Work out the finished part from the listing and answer in its coordinate system (mm). A direction names the side the tool comes from. Coordinates: 2 decimals unless noted, no trailing zeros. Order: outer loops, then holes, each group sorted by start corner. A loop starts at its lowest first (then second) coordinate and runs counter-clockwise, first axis right, second up. Notation, with made-up numbers: M -16,4.5 L 11,4.5 A27 cw 11,32.5 Z; hole C -6,81 d8. An arc over 180 degrees is marked long. Answer in a Markdown table with one row per item. Add a question column.
Item 1: The mould has two halves that part along X. Classify faces 3 (the face through (-10.79, 46, 1.24)), 4 (the face through (-10.91, 46.94, 2.96)), 5 (the face through (-11.246, 34.387, 0.246)), 6 (the face through (-13, 46, 6)): released by +X, released by -X, zero draft, split by the parting line, or undercut.
Item 2: The part is cut by section D-D (z = 0.85). Write down the section's boundary in (x, y), then the cut area to 3 significant figures.
Item 3: Consider line 1 (Y direction, x = -10, z = 3.65); line 2 (Y direction, x = -10, z = 0.3); line 3 (X direction, y = 35.75, z = 2.45). Determine where each line is inside the solid, lowest interval first. Write a range as from..to.
Item 4: The part is cut by section A-A (x = -10). Write down the section's boundary in (y, z).
Item 5: Flat-ended cylindrical pins translate along their axes: pin 1 Ø7 at (x, y) = (-10, 40) entering from -Z (3 decimals); pin 2 Ø1.5 at (x, z) = (-11.5, 2.5) entering from +Y; pin 3 Ø1 at (y, z) = (44, 2) entering from +X; pin 4 Ø1.5 at (x, y) = (-14.5, 42.5) entering from +Z. Find the tip coordinate at first contact, or state that the pin passes through.
Item 6: Which of the six approach directions +Z, -Z, +X, -X, +Y, -Y give full straight-line access (tool end or side, diameter ignored) to faces 1 (the face through (-10.8, 46.2, 4)), 2 (the face through (-11, 46, 0))?
Item 7: The part is cut by section C-C (z = 4.3). Write down the section's boundary in (x, y).
Item 8: The part is cut by section B-B (y = 40). Write down the section's boundary in (x, z).
from build123d import *

# Parameters (mm, degrees)
CYLINDER011_R     = 6.25
CYLINDER011_DEPTH = 10
CYLINDER010_R     = 6.05
CYLINDER010_DEPTH = 10
CYLINDER009_R     = 5.75
CYLINDER009_DEPTH = 10
CYLINDER008_R     = 7
CYLINDER008_DEPTH = 6


with BuildPart() as bluetmp06:
    # Cylinder011 → Cylinder011 (new body)
    with BuildSketch(Plane.XY.offset(2)):
        Circle(CYLINDER011_R)
    extrude(amount=CYLINDER011_DEPTH)


with BuildPart() as bluetmp04:
    # Cylinder010 → Cylinder010 (new body)
    with BuildSketch(Plane.XY.offset(0.5)):
        Circle(CYLINDER010_R)
    extrude(amount=CYLINDER010_DEPTH)


with BuildPart() as bluetmp02:
    # Cylinder009 → Cylinder009 (new body)
    with BuildSketch(Plane.XY):
        Circle(CYLINDER009_R)
    extrude(amount=CYLINDER009_DEPTH)


with BuildPart() as blueholder:
    # Cylinder008 → Cylinder008 (new body)
    with BuildSketch(Plane.XY):
        Circle(CYLINDER008_R)
    extrude(amount=CYLINDER008_DEPTH)

    # Cut005: cut BlueTmp02
    add(bluetmp02.part, mode=Mode.SUBTRACT)

    # Cut006: cut BlueTmp04
    add(bluetmp04.part, mode=Mode.SUBTRACT)

    # Cut007: cut BlueTmp06
    add(bluetmp06.part, mode=Mode.SUBTRACT)


with BuildPart() as blueholder_1:
    # Cut007 placement: moved
    add(blueholder.part.moved(Location((-10, 40, 0))))


solid = blueholder_1.part
Reply:
| question | item | result |
|---|---|---|
| 1 | face 3 | undercut |
| 1 | face 4 | split by the parting line |
| 1 | face 5 | undercut |
| 1 | face 6 | zero draft |
| 2 | outline | C -10,40 d14; hole C -10,40 d12.1 |
| 2 | area | 38.9 mm2 |
| 3 | line 1 | y = 33..33.75, 46.25..47 |
| 3 | line 2 | y = 33..34.25, 45.75..47 |
| 3 | line 3 | x = -15.56..-14.58, -5.42..-4.44 |
| 4 | outline | M 33,0 L 34.25,0 L 34.25,0.5 L 33.95,0.5 L 33.95,2 L 33.75,2 L 33.75,6 L 33,6 Z; M 45.75,0 L 47,0 L 47,6 L 46.25,6 L 46.25,2 L 46.05,2 L 46.05,0.5 L 45.75,0.5 Z |
| 5 | pin 1 | passes through |
| 5 | pin 2 | stops at y = 46.96 |
| 5 | pin 3 | stops at x = -3.94 |
| 5 | pin 4 | stops at z = 0.5 |
| 6 | face 1 | +Z |
| 6 | face 2 | -Z, +X, -X, +Y, -Y |
| 7 | outline | C -10,40 d14; hole C -10,40 d12.5 |
| 8 | outline | M -17,0 L -15.75,0 L -15.75,0.5 L -16.05,0.5 L -16.05,2 L -16.25,2 L -16.25,6 L -17,6 Z; M -4.25,0 L -3,0 L -3,6 L -3.75,6 L -3.75,2 L -3.95,2 L -3.95,0.5 L -4.25,0.5 Z |
